Check sheet for the modelled part. Datum: model origin and axes. Units: mm. A direction names the side the tool comes from. Give positions to 0.01 mm unless a question says otherwise; leave off trailing zeros. Loops run counter-clockwise (first coordinate to the right, second up) from the corner with the lowest first, then second, coordinate; pieces in that order, holes last. Notation, with made-up numbers: (4.25, 54) -> (9.25, 54) arc R32 cw to (9.25, 90) -> close; hole circle Ø2 at (1.5, 6). An arc over 180 degrees is marked (long way). Write each question's results on one line, items separated by ' | '. Start each with the question number.
Item 1: Mould release check, pull along X, two halves, no side actions. Record for faces 6 (the face through (14.985, 328.85, 0.66)), 7 (the face through (0, -20, 38.5)), 8 (the face through (15, -19, -1)), 9 (the face through (-15, -19, -1)): pulls with the +X half, pulls with the -X half, needs draft (parallel to the pull), parting line crosses it, or undercut.
Item 2: Access from +Z, -Z, +X, -X, +Y, -Y to the whole of each face (thin tool, end or side, straight path). Record for faces 1 (the face through (24, 0, 0)), 2 (the face through (0, -20, -38.5)), 3 (the face through (-24, 0, 0)), 4 (the face through (0, -70, 0)), 5 (the face through (0, 50, 0)).
Item 3: Scan lines: line 1 along Z through (x, y) = (-1.5, 101); line 2 along Z through (x, y) = (0, 285); line 3 along Y through (x, z) = (2, 12). Record each from-to range of solid material in increasing order.
Item 4: Cross-section at A-A on z = 0. Enter the section's corners in (x, y).
Item 5: Cross-section at D-D on z = 27. Enter the section's corners in (x, y), then the cut area to 3 significant figures.
Item 6: Cross-section at B-B on x = -6.5. Enter the section's corners in (y, z).
Item 7: Gauge pin test, flat ends, axial feed: pin 1 Ø1.5 at (x, z) = (-9, 37.5) entering from +Y; pin 2 Ø9 at (x, z) = (-5.5, -6.5) entering from +Y; pin 3 Ø3 at (x, y) = (9, 59.5) entering from -Z; pin 4 Ø18 at (y, z) = (-37.34, 0) entering from -X. Record the tip position at first contact, or that the pin passes through.
Item 8: Cross-section at C-C on y = 72.5. Enter the section's corners in (x, z), then the cut area to 3 significant figures.
from build123d import *

# Parameters (mm, degrees)
F0_R     = 38.5
F1_DEPTH = 600
F2_W     = 30
F2_H     = 77
F3_DEPTH = 70
F4_R     = 15
F5_DEPTH = 53.501
F6_R     = 30
F7_R     = 15
F8_DEPTH = 550


with BuildPart() as f1:
    # F0 (on Front) → F1 (new body)
    with BuildSketch(Plane.XZ):
        Circle(F0_R)
    extrude(amount=-F1_DEPTH)

    # F2 (on face) → F3 (join)
    with BuildSketch(Plane.XZ):
        Rectangle(F2_W, F2_H)
    extrude(amount=F3_DEPTH)

    # F4 (on face) → F5 (cut, through all)
    with BuildSketch(Plane.YZ.offset(15)):
        with Locations((-37.336115, 0)):
            Circle(F4_R)
    extrude(amount=-F5_DEPTH, mode=Mode.SUBTRACT)

    # F6
    f6_edges = [f1.edges().sort_by_distance(p)[0] for p in [
        (0, -70, 38.5),
        (0, -70, -38.5),
    ]]
    fillet(f6_edges, radius=F6_R)

    # F7 (on face) → F8 (cut)
    with BuildSketch(Plane(origin=(0, 600, 0), x_dir=(-1, 0, 0), z_dir=(0, 1, 0))):
        Circle(F7_R)
    extrude(amount=-F8_DEPTH, mode=Mode.SUBTRACT)


solid = f1.part
Answer sheet:
1) face 6: undercut | face 7: needs draft | face 8: pulls with the +X half | face 9: pulls with the -X half
2) face 1: +Z, -Z, +X, -Y | face 2: -Z, +X, -X, +Y, -Y | face 3: +Z, -Z, -X, -Y | face 4: +Z, -Z, +X, -X, -Y | face 5: +Y
3) line 1: z = -38.47 to -14.92, 14.92 to 38.47 | line 2: z = -38.5 to -15, 15 to 38.5 | line 3: y = -69.8 to -46.34, -28.34 to 50
4) outline: (-38.5, 0) -> (-15, 0) -> (-15, -22.34) -> (15, -22.34) -> (15, 0) -> (38.5, 0) -> (38.5, 600) -> (15, 600) -> (15, 50) -> (-15, 50) -> (-15, 600) -> (-38.5, 600) -> close; (-15, -70) -> (15, -70) -> (15, -52.34) -> (-15, -52.34) -> close
5) outline: (-27.45, 0) -> (-15, 0) -> (-15, -63.62) -> (15, -63.62) -> (15, 0) -> (27.45, 0) -> (27.45, 600) -> (-27.45, 600) -> close | area: 34,800 mm²
6) outline: (-70, -8.5) arc R30 ccw to (-40, -38.5) -> (0, -38.5) -> (0, -37.95) -> (600, -37.95) -> (600, -13.52) -> (50, -13.52) -> (50, 13.52) -> (600, 13.52) -> (600, 37.95) -> (0, 37.95) -> (0, 38.5) -> (-40, 38.5) arc R30 ccw to (-70, 8.5) -> close; hole circle Ø30 at (-37.34, 0)
7) pin 1: stops at y = 600 | pin 2: stops at y = 50 | pin 3: stops at z = -37.76 | pin 4: passes through
8) outline: circle Ø77 at (0, 0); hole circle Ø30 at (0, 0) | area: 3,950 mm²
